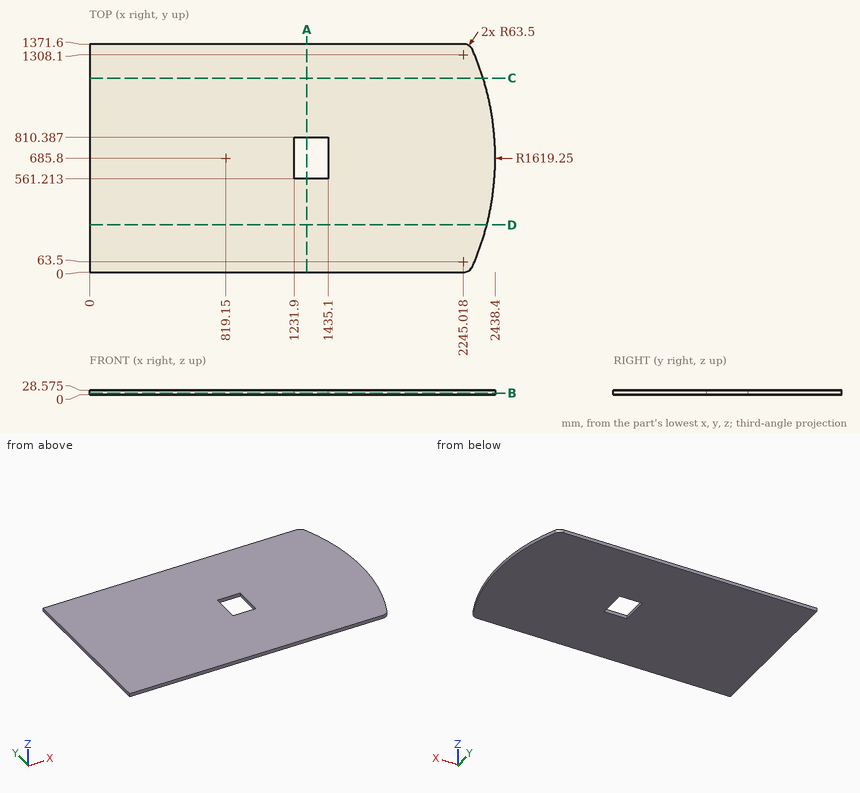
Print and shaded views of the part. All mm, measured from the part's lowest x, y and z. Give positions to 0.01 mm unless a question says otherwise; leave off trailing zeros. Write each loop counter-clockwise with the first axis right and the second up, starting at its lowest first coordinate (ties: lowest second). Pieces come first, ordered by that corner, then holes. Notation, with made-up numbers: M -3.5,-0.5 L 31.5,-0.5 A26 ccw 31.5,32.5 Z; hole C 8.5,-39.75 d5. An arc over 180 degrees is marked long. Use a Markdown table: item, result.
1) Cut at D-D (y = 285). List the corners of the cut face in (x, z) (1 decimal).
Responses:
| item | result |
|---|---|
| outline | M 0,0 L 2388,0 L 2388,28.6 L 0,28.6 Z |
2) Drill centre lines: line 1 (X direction, y = 669, z = 13); line 2 (X direction, y = 660, z = 8) (1 decimal); line 3 (X direction, y = 947, z = 12.25) (1 decimal). Where is each one in solid material? Low to high. Write a range as from..to.
Responses:
| item | result |
|---|---|
| line 1 | x = 0..1231.9, 1435.1..2438.31 |
| line 2 | x = 0..1231.9, 1435.1..2438.2 |
| line 3 | x = 0..2417.2 |
3) Cut at A-A (x = 1306). List the corners of the cut face in (y, z) (1 decimal), and give its area (3 significant figures).
Responses:
| item | result |
|---|---|
| outline | M 0,0 L 561.2,0 L 561.2,28.6 L 0,28.6 Z; M 810.4,0 L 1371.6,0 L 1371.6,28.6 L 810.4,28.6 Z |
| area | 32,100 mm2 |
4) Pin check, flat tips, straight feed: pin 1 (5 mm diameter, centred on y = 173, z = 13, fed in from +X); pin 2 (12 mm diameter, centred on y = 973, z = 23.5, fed in from -X); pin 3 (2 mm diameter, centred on y = 496, z = 7.5, fed in from +X) (1 decimal). Stop position of each tip, or through.
Responses:
| item | result |
|---|---|
| pin 1 | stops at x = 2355.89 |
| pin 2 | stops at x = 0 |
| pin 3 | stops at x = 2427.4 |
5) Cut at C-C (y = 1167). List the corners of the cut face in (x, z) (1 decimal).
Responses:
| item | result |
|---|---|
| outline | M 0,0 L 2365.2,0 L 2365.2,28.6 L 0,28.6 Z |
6) Cut at B-B (z = 10.75). List the corners of the cut face in (x, y).
Responses:
| item | result |
|---|---|
| outline | M 0,0 L 2245.02,0 A63.5 ccw 2303.22,38.1 A1619.25 ccw 2303.22,1333.5 A63.5 ccw 2245.02,1371.6 L 0,1371.6 Z; hole M 1231.9,561.21 L 1435.1,561.21 L 1435.1,810.39 L 1231.9,810.39 Z |
